For this review, take the finished solid that the model builds, in its own axes (mm). A direction names the side the tool comes from. Give positions to 0.01 mm unless a question says otherwise; leave off trailing zeros. Loops run counter-clockwise (first coordinate to the right, second up) from the corner with the lowest first, then second, coordinate; pieces in that order, holes last. Notation, with made-up numbers: (48.25, -37) - (73.25, -37) arc R20 ccw to (73.25, -13) - close; hole circle Ø2 at (73, 41). An arc over 180 degrees is marked (long way). Answer in a Markdown table with one row per item.
```python
from build123d import *

# Parameters (mm, degrees)
BOSS_EXTRUDE1_DEPTH      = 10
BOSS_EXTRUDE1_DEPTH_BACK = 10


# Read off the part's stored shape, not the designer's step: Hole1
with BuildPart() as part:
    # Sketch1 → Boss-Extrude1 (new, two sides: drawn at the far end of the back side and taken through both)
    with BuildSketch(Plane(origin=(0, 0, 0), x_dir=(1, 0, 0), z_dir=(0, 1, 0)).offset(-BOSS_EXTRUDE1_DEPTH_BACK)):
        Polygon((41.092590889, 58.060996062), (-38.907409111, 58.060996062), (-38.907409111, 43.060996062), (-18.907409111, 43.060996062), (-18.907409111, 28.060996062), (-38.907409111, 28.060996062), (-38.907409111, 13.060996062), (-13.907409111, 13.060996062), (-13.907409111, 3.060996062), (-38.907409111, 3.060996062), (-38.907409111, -11.939003938), (-18.907409111, -11.939003938), (-18.907409111, -26.939003938), (-38.907409111, -26.939003938), (-38.907409111, -41.939003938), (41.092590889, -41.939003938), (41.092590889, -26.939003938), (21.092590889, -26.939003938), (21.092590889, -11.939003938), (41.092590889, -11.939003938), (41.092590889, 3.060996062), (16.092590889, 3.060996062), (16.092590889, 13.060996062), (41.092590889, 13.060996062), (41.092590889, 28.060996062), (21.092590889, 28.060996062), (21.092590889, 43.060996062), (41.092590889, 43.060996062), align=None)
    extrude(amount=BOSS_EXTRUDE1_DEPTH + BOSS_EXTRUDE1_DEPTH_BACK)

    # Hole1 outline → Hole1 (revolve, cut)
    with BuildSketch(Plane(origin=(28.620361889, -0.784426919, 0), x_dir=(1, 0, 0), z_dir=(0, -1, 0))):
        Polygon((5, 41.939003938), (0, 41.939003938), (0, 26.939003938), (4.476188458, 26.939003938), align=None)
        Polygon((3.428565373, -3.060996062), (3.952376915, 11.939003938), (0, 11.939003938), (0, -3.060996062), align=None)
        Polygon((2.555546136, -28.060996062), (3.079357678, -13.060996062), (0, -13.060996062), (0, -28.060996062), align=None)
        Polygon((1.507923051, -58.060996062), (2.031734593, -43.060996062), (0, -43.060996062), (0, -58.060996062), align=None)
    revolve(axis=Axis((28.620361889, -0.784426919, 0), (0, 0, 1)), mode=Mode.SUBTRACT)


solid = part.part
```
1. Clearance check with flat-ended pins moving along their axes: pin 1 (2 mm diameter, centred on y = 0.5, z = -38, fed in from +X); pin 2 (12 mm diameter, centred on y = 2.5, z = 18, fed in from -X); pin 3 (5 mm diameter, centred on y = -0.5, z = -7.5, fed in from -X). State where each tip first meets the part, or that it passes through.
Values:
| item | result |
|---|---|
| pin 1 | stops at x = 21.09 |
| pin 2 | stops at x = -18.91 |
| pin 3 | stops at x = -13.91 |
2. We need section B-B, the plane x = -20. Give the boundary of the cut face in (y, z), and give its area (3 significant figures).
Values:
| item | result |
|---|---|
| outline | (-10, -58.06) - (10, -58.06) - (10, -43.06) - (-10, -43.06) - close; (-10, -28.06) - (10, -28.06) - (10, -13.06) - (-10, -13.06) - close; (-10, -3.06) - (10, -3.06) - (10, 11.94) - (-10, 11.94) - close; (-10, 26.94) - (10, 26.94) - (10, 41.94) - (-10, 41.94) - close |
| area | 1,200 mm^2 |
3. Wall thickness on line 1 (Z direction, x = 35.5, y = -4.25); line 2 (Z direction, x = -17.5, y = -5.5); line 3 (X direction, y = 3, z = -41): over which ranges is each line inside the solid? List them lowest first. Write a range as [from, to].
Values:
| item | result |
|---|---|
| line 1 | z = [-58.06, -43.06], [-28.06, -13.06], [-3.06, 11.94], [26.94, 41.94] |
| line 2 | z = [-58.06, -13.06], [-3.06, 41.94] |
| line 3 | x = [-18.91, 21.09] |
4. We need section C-C, the plane y = -8.5. Give the boundary of the cut face in (x, z).
Values:
| item | result |
|---|---|
| outline | (-38.91, -58.06) - (41.09, -58.06) - (41.09, -43.06) - (21.09, -43.06) - (21.09, -28.06) - (41.09, -28.06) - (41.09, -13.06) - (16.09, -13.06) - (16.09, -3.06) - (41.09, -3.06) - (41.09, 11.94) - (21.09, 11.94) - (21.09, 26.94) - (41.09, 26.94) - (41.09, 41.94) - (-38.91, 41.94) - (-38.91, 26.94) - (-18.91, 26.94) - (-18.91, 11.94) - (-38.91, 11.94) - (-38.91, -3.06) - (-13.91, -3.06) - (-13.91, -13.06) - (-38.91, -13.06) - (-38.91, -28.06) - (-18.91, -28.06) - (-18.91, -43.06) - (-38.91, -43.06) - close |
5. We need section D-D, the plane z = -40. Give the boundary of the cut face in (x, y).
Values:
| item | result |
|---|---|
| outline | (-18.91, -10) - (21.09, -10) - (21.09, 10) - (-18.91, 10) - close |
6. Mouldability with a two-part tool opening along Z and no side actions: class faces 4 (the face through (26, 2, -13.061)), 5 (the face through (-26, 0, -3.061)), 6 (the face through (33, -2.6, 34.5)), 7 (the face through (41.093, 0, 35)) as released by +Z, released by -Z, zero draft, split by the parting line, or undercut.
Values:
| item | result |
|---|---|
| face 4 | undercut |
| face 5 | undercut |
| face 6 | released by +Z |
| face 7 | zero draft |
7. For faces 1 (the face through (-18.907, 0, 19)), 2 (the face through (30.31, -0.25, -50.46)), 3 (the face through (21.093, 0, -35)), list the 3-axis set-ups (+Z, -Z, +X, -X, +Y, -Y) from which the entire face can be reached by the end or side of a thin tool; tool diameter is ignored.
Values:
| item | result |
|---|---|
| face 1 | -X, +Y, -Y |
| face 2 | +Z |
| face 3 | +X, +Y, -Y |
8. We need section A-A, the plane x = 18. Give the boundary of the cut face in (y, z).
Values:
| item | result |
|---|---|
| outline | (-10, -58.06) - (10, -58.06) - (10, -13.06) - (-10, -13.06) - close; (-10, -3.06) - (10, -3.06) - (10, 41.94) - (-10, 41.94) - close |
